from build123d import *

# Parameters (mm, degrees)
SKETCH1_R           = 24
SKETCH1_R_2         = 1.65
SKETCH1_W           = 5.5
SKETCH1_H           = 10.5
BOSS_EXTRUDE1_DEPTH = 3
SKETCH2_R           = 12
SKETCH2_R_2         = 1.65
SKETCH2_W           = 5.5
SKETCH2_H           = 10.5
BOSS_EXTRUDE2_DEPTH = 1
SKETCH4_R           = 10
SKETCH4_R_2         = 1.65
SKETCH4_W           = 5.5
SKETCH4_H           = 10.5
BOSS_EXTRUDE3_DEPTH = 7.2


with BuildPart() as part:
    # Sketch1 → Boss-Extrude1 (new body)
    with BuildSketch(Plane(origin=(0, 0, 0), x_dir=(1, 0, 0), z_dir=(0, 1, 0))):
        Circle(SKETCH1_R)
        with Locations((-6, 0)):
            Circle(SKETCH1_R_2, mode=Mode.SUBTRACT)
        with Locations((6, 0)):
            Circle(SKETCH1_R_2, mode=Mode.SUBTRACT)
        Rectangle(SKETCH1_W, SKETCH1_H, mode=Mode.SUBTRACT)
    extrude(amount=BOSS_EXTRUDE1_DEPTH)

    # Sketch2 → Boss-Extrude2 (add)
    with BuildSketch(Plane(origin=(0, 3, 0), x_dir=(1, 0, 0), z_dir=(0, 1, 0))):
        with Locations((0, 2)):
            Circle(SKETCH2_R)
        with Locations((-6, 0)):
            Circle(SKETCH2_R_2, mode=Mode.SUBTRACT)
        with Locations((6, 0)):
            Circle(SKETCH2_R_2, mode=Mode.SUBTRACT)
        Rectangle(SKETCH2_W, SKETCH2_H, mode=Mode.SUBTRACT)
    extrude(amount=BOSS_EXTRUDE2_DEPTH)

    # Sketch4 → Boss-Extrude3 (add)
    with BuildSketch(Plane(origin=(0, 4, 0), x_dir=(1, 0, 0), z_dir=(0, 1, 0))):
        with Locations((0, 2)):
            Circle(SKETCH4_R)
        with Locations((-6, 0)):
            Circle(SKETCH4_R_2, mode=Mode.SUBTRACT)
        with Locations((6, 0)):
            Circle(SKETCH4_R_2, mode=Mode.SUBTRACT)
        Rectangle(SKETCH4_W, SKETCH4_H, mode=Mode.SUBTRACT)
    extrude(amount=BOSS_EXTRUDE3_DEPTH)


solid = part.part
Can you work these out from the model? Positions are in its coordinate system, mm. A direction names the side the tool comes from. Round coordinates to 2 decimals unless told otherwise and drop trailing zeros. Write each loop counter-clockwise with the first axis right and the second up, starting at its lowest first coordinate (ties: lowest second). Pieces come first, ordered by that corner, then holes. Notation, with made-up numbers: M 27,-21.5 L 80,-21.5 A25 ccw 80,14.5 Z; hole C 54,-1 d10. An arc over 180 degrees is marked long. Use CSV: the item, a comma, the result in double quotes.
(1) We'd pull the mould along Z, two halves only. Please class faces 4 (the cylindrical face through (-23.977, 1.479, -1.055)), 5 (the flat face through (2.75, 6, 0)), 6 (the flat face through (4, 11.2, -2)), 7 (the flat face through (0, 6, -5.25)): +Z half, -Z half, draft (parallel to the pull), parting line (faces both ways), or undercut.
Check values:
face 4,"parting line"
face 5,"undercut"
face 6,"draft"
face 7,"undercut"
(2) I need wall thicknesses on line 1 along X through (y, z) = (4.25, 0); line 2 along X through (y, z) = (3.5, 0); line 3 along Z through (x, y) = (-5.5, 10). Which ranges of each line are inside material? Lowest first, please.
Check values:
line 1,"-9.8 to -7.65, -4.35 to -2.75, 2.75 to 4.35, 7.65 to 9.8"
line 2,"-11.83 to -7.65, -4.35 to -2.75, 2.75 to 4.35, 7.65 to 11.83"
line 3,"-10.35 to -1.57, 1.57 to 6.35"
(3) Imagine slicing it at B-B (z = 1). Write out the boundary of the cut face in (x, y).
Check values:
outline,"M -23.98,0 L -7.31,0 L -7.31,11.2 L -9.54,11.2 L -9.54,4 L -11.62,4 L -11.62,3 L -23.98,3 Z; M -4.69,0 L -2.75,0 L -2.75,11.2 L -4.69,11.2 Z; M 2.75,0 L 4.69,0 L 4.69,11.2 L 2.75,11.2 Z; M 7.31,0 L 23.98,0 L 23.98,3 L 11.62,3 L 11.62,4 L 9.54,4 L 9.54,11.2 L 7.31,11.2 Z"
(4) On a 3-axis mill with a long thin cutter (end or side, diameter ignored), from which of +Z, -Z, +X, -X, +Y, -Y can I reach the whole of each face in a straight line? I mean faces 1 (the cylindrical face through (-11.99, 3.49, -2.53)), 2 (the flat face through (-2.75, 6, 0)), 3 (the flat face through (0, 0, -6)). Say none if no direction works.
Check values:
face 1,"+Y"
face 2,"+Y, -Y"
face 3,"+Z, -Z, +X, -X, -Y"
(5) Imagine slicing it at A-A (x = 0). Write out the boundary of the cut face in (y, z).
Check values:
outline,"M 0,-24 L 3,-24 L 3,-14 L 4,-14 L 4,-12 L 11.2,-12 L 11.2,-5.25 L 0,-5.25 Z; M 0,5.25 L 11.2,5.25 L 11.2,8 L 4,8 L 4,10 L 3,10 L 3,24 L 0,24 Z"
(6) Imagine slicing it at D-D (z = -8). Write out the boundary of the cut face in (x, y), plus the area to 3 significant figures.
Check values:
outline,"M -22.63,0 L 22.63,0 L 22.63,3 L 10.39,3 L 10.39,4 L 8,4 L 8,11.2 L -8,11.2 L -8,4 L -10.39,4 L -10.39,3 L -22.63,3 Z"
area,"272 mm^2"
(7) Imagine slicing it at C-C (y = 1.25). Write out the boundary of the cut face in (x, z), plus the area to 3 significant figures.
Check values:
outline,"C 0,0 d48; hole C -6,0 d3.3; hole M -2.75,-5.25 L 2.75,-5.25 L 2.75,5.25 L -2.75,5.25 Z; hole C 6,0 d3.3"
area,"1,730 mm^2"
(8) I'm going to push flat-ended pins straight in: pin 1 (1 mm diameter, centred on y = 6, z = -5.5, fed in from -X); pin 2 (4 mm diameter, centred on x = -14, y = 2, fed in from -Z); pin 3 (4.5 mm diameter, centred on x = -1, y = 3, fed in from +Z); pin 4 (2 mm diameter, centred on x = -6, z = 0, fed in from -Y). Where does each tip first touch, or does it pass through?
Check values:
pin 1,"x = -9.54"
pin 2,"z = -20.78"
pin 3,"z = 24"
pin 4,"through"
